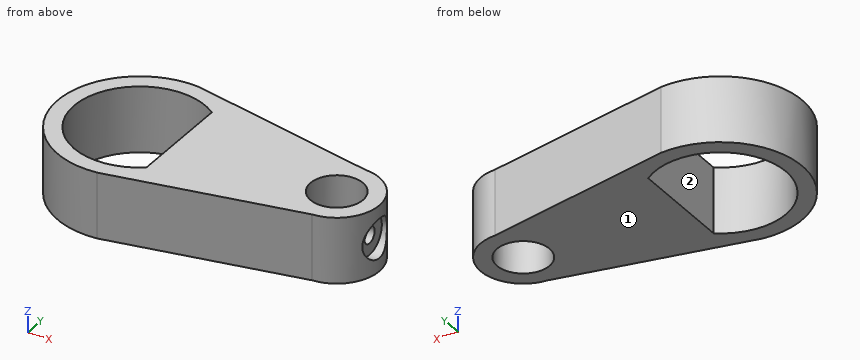
```python
from build123d import *

# Parameters (mm, degrees)
SKETCH1_R           = 4
BOSS_EXTRUDE1_DEPTH = 10
CUT_EXTRUDE1_DEPTH  = 7
SKETCH3_R           = 3
CUT_EXTRUDE2_DEPTH  = 2


with BuildPart() as part:
    # Sketch1 → Boss-Extrude1 (new body)
    with BuildSketch(Plane.XY):
        with BuildLine():
            Line((15.283584765, 6.493810875), (-13.726969973, 12.435006817))
            ThreePointArc((-13.726969973, 12.435006817), (-27.5, 0), (-13.726969973, -12.435006817))
            Line((-13.726969973, -12.435006817), (15.283584765, -6.493810875))
            ThreePointArc((15.283584765, -6.493810875), (21.5, 0), (15.283584765, 6.493810875))
        make_face()
        with Locations((15, 0)):
            Circle(SKETCH1_R, mode=Mode.SUBTRACT)
        with BuildLine():
            Line((-9, -8), (-9, 8))
            ThreePointArc((-9, 8), (-25, 0), (-9, -8))
        make_face(mode=Mode.SUBTRACT)
    extrude(amount=BOSS_EXTRUDE1_DEPTH)

    # Sketch2 → Cut-Extrude1 (cut)
    with BuildSketch(Plane(origin=(22, 0, 0), x_dir=(0, 0, -1), z_dir=(1, 0, 0))):
        with BuildLine():
            ThreePointArc((-6.25, 0), (-5, -1.25), (-3.75, 0))
            Line((-3.75, 0), (-6.25, 0))
        make_face()
        with BuildLine():
            Line((-6.25, 0), (-3.75, 0))
            ThreePointArc((-3.75, 0), (-5, 1.25), (-6.25, 0))
        make_face()
    extrude(amount=-CUT_EXTRUDE1_DEPTH, mode=Mode.SUBTRACT)

    # Sketch3 → Cut-Extrude2 (cut)
    with BuildSketch(Plane(origin=(22, 0, 0), x_dir=(0, 0, -1), z_dir=(1, 0, 0))):
        with Locations((-5, 0)):
            Circle(SKETCH3_R)
    extrude(amount=-CUT_EXTRUDE2_DEPTH, mode=Mode.SUBTRACT)


solid = part.part
```
The model under review builds one solid part; all positions refer to its coordinate system, in mm. Face numbers are marked on the shaded views. A direction names the side the tool comes from. Give positions to 0.01 mm unless a question says otherwise; leave off trailing zeros. Write each loop counter-clockwise with the first axis right and the second up, starting at its lowest first coordinate (ties: lowest second). Pieces come first, ordered by that corner, then holes.
(1) Consider section B-B, the plane x = -15. Give the boundary of the cut face in (y, z).
(2) Tool access review of the marked faces 1 and 2: name each direction out of +Z, -Z, +X, -X, +Y, -Y from which nothing blocks a thin tool from reaching the whole face with its end or side.
(3) Consider section D-D, the plane y = 5.5. Give the boundary of the cut face in (x, z).
(4) For P1, Ø2, axis at y = -7.5, z = 7, coming from the -X side; P2, Ø3.5, axis at y = 0, z = 5, coming from the +X side; P3, Ø1.5, axis at y = 2.5, z = 1.5, coming from the -X side, all flat-tipped, find the tip position at first contact; note any pin that passes through.
(5) Consider section A-A, the plane y = 0. Give the boundary of the cut face in (x, z), and give its area (4 significant figures).
(6) Consider section C-C, the plane z = 2.5. Give the boundary of the cut face in (x, y) (3 decimals).
(7) To check wall thickness, follow L1, parallel to Z at x = 20.8, y = 0; L2, parallel to Y at x = -15, z = 2.75; L3, parallel to X at y = -2.25, z = 6.25. State the ranges of each line that lie inside material, in increasing order.
Returned:
1. outline: (-12.5, 0) - (-10, 0) - (-10, 10) - (-12.5, 10) - close; (10, 0) - (12.5, 0) - (12.5, 10) - (10, 10) - close
2. face 1: -Z, +X, -X, +Y, -Y
2. face 2: +Z, -Z
3. outline: (-26.22, 0) - (-23.35, 0) - (-23.35, 10) - (-26.22, 10) - close; (-9, 0) - (18.46, 0) - (18.46, 10) - (-9, 10) - close
4. P1: stops at x = -25.68
4. P2: stops at x = 20
4. P3: stops at x = -27.38
5. outline: (-27.5, 0) - (-25, 0) - (-25, 10) - (-27.5, 10) - close; (-9, 0) - (11, 0) - (11, 10) - (-9, 10) - close; (19, 0) - (21.5, 0) - (21.5, 2) - (20, 2) - (20, 3.75) - (19, 3.75) - close; (19, 6.25) - (20, 6.25) - (20, 8) - (21.5, 8) - (21.5, 10) - (19, 10) - close
5. area: 238.5 mm2
6. outline: (-13.727, -12.435) - (15.284, -6.494) arc R6.5 ccw to (21.285, -1.658) - (20, -1.658) - (20, 1.658) - (21.285, 1.658) arc R6.5 ccw to (15.284, 6.494) - (-13.727, 12.435) arc R12.5 ccw (long way) to start; hole (-9, -8) - (-9, 8) arc R10 ccw (long way) to start; hole circle Ø8 at (15, 0)
7. L1: z = 0 to 2, 8 to 10
7. L2: y = -12.5 to -10, 10 to 12.5
7. L3: x = -27.3 to -24.74, -9 to 11.69, 18.31 to 20
